The model under review builds one solid part; all positions refer to its coordinate system, in mm. A direction names the side the tool comes from. Round coordinates to 2 decimals unless told otherwise and drop trailing zeros. Write each loop counter-clockwise with the first axis right and the second up, starting at its lowest first coordinate (ties: lowest second). Pieces come first, ordered by that corner, then holes. Notation, with made-up numbers: (30, 4.25) - (64, 4.25) arc R25 ccw to (64, 27.25) - close; hole circle Ø7 at (65.5, 42). An arc over 180 degrees is marked (long way). Return JSON: item names as keys, results as strings.
from build123d import *

# Parameters (mm, degrees)
BOSS_EXTRUDE1_DEPTH = 3
SKETCH2_R           = 17
BOSS_EXTRUDE2_DEPTH = 5.5
SKETCH5_R           = 14
BOSS_EXTRUDE3_DEPTH = 3.5
SKETCH6_R           = 11
CUT_EXTRUDE1_DEPTH  = 44.5
SKETCH7_R           = 2.5
CUT_EXTRUDE2_DEPTH  = 44.5
SKETCH8_R           = 2.5
CUT_EXTRUDE3_DEPTH  = 44.5
SKETCH9_R           = 2.5
CUT_EXTRUDE4_DEPTH  = 44.5
SKETCH10_R          = 2.5
CUT_EXTRUDE5_DEPTH  = 44.5
FILLET23_R          = 2


with BuildPart() as part:
    # Sketch1 → Boss-Extrude1 (new body)
    with BuildSketch(Plane(origin=(0, 0, 0), x_dir=(1, 0, 0), z_dir=(0, 1, 0))):
        with BuildLine():
            ThreePointArc((-12.368882592, -22.86942814), (-2.248386141, -25.902601409), (8.243375366, -24.65860423))
            ThreePointArc((8.243375366, -24.65860423), (11.092172188, -24.325815059), (13.835297391, -25.163464204))
            ThreePointArc((13.835297391, -25.163464204), (20.585915101, -24.499389777), (22.403221797, -17.964159812))
            ThreePointArc((22.403221797, -17.964159812), (22.050754674, -15.117730664), (22.86942814, -12.368882592))
            ThreePointArc((22.86942814, -12.368882592), (25.902601409, -2.248386141), (24.65860423, 8.243375366))
            ThreePointArc((24.65860423, 8.243375366), (24.325815059, 11.092172188), (25.163464204, 13.835297391))
            ThreePointArc((25.163464204, 13.835297391), (24.499389777, 20.585915101), (17.964159812, 22.403221797))
            ThreePointArc((17.964159812, 22.403221797), (15.117730664, 22.050754674), (12.368882592, 22.86942814))
            ThreePointArc((12.368882592, 22.86942814), (2.248386141, 25.902601409), (-8.243375366, 24.65860423))
            ThreePointArc((-8.243375366, 24.65860423), (-11.092172188, 24.325815059), (-13.835297391, 25.163464204))
            ThreePointArc((-13.835297391, 25.163464204), (-20.585915101, 24.499389777), (-22.403221797, 17.964159812))
            ThreePointArc((-22.403221797, 17.964159812), (-22.050754674, 15.117730664), (-22.86942814, 12.368882592))
            ThreePointArc((-22.86942814, 12.368882592), (-25.902601409, 2.248386141), (-24.65860423, -8.243375366))
            ThreePointArc((-24.65860423, -8.243375366), (-24.325815059, -11.092172188), (-25.163464204, -13.835297391))
            ThreePointArc((-25.163464204, -13.835297391), (-24.499389777, -20.585915101), (-17.964159812, -22.403221797))
            ThreePointArc((-17.964159812, -22.403221797), (-15.117730664, -22.050754674), (-12.368882592, -22.86942814))
        make_face()
    extrude(amount=-BOSS_EXTRUDE1_DEPTH)

    # Sketch2 → Boss-Extrude2 (add)
    with BuildSketch(Plane(origin=(0, 0, 0), x_dir=(1, 0, 0), z_dir=(0, 1, 0))):
        with Locations(Location((0, 0, 0), (0, 0, 270))):
            Circle(SKETCH2_R)
    extrude(amount=BOSS_EXTRUDE2_DEPTH)

    # Sketch5 → Boss-Extrude3 (add)
    with BuildSketch(Plane(origin=(0, 5.5, 0), x_dir=(1, 0, 0), z_dir=(0, 1, 0))):
        with Locations(Location((0, 0, 0), (0, 0, 270))):
            Circle(SKETCH5_R)
    extrude(amount=BOSS_EXTRUDE3_DEPTH)

    # Sketch6 → Cut-Extrude1 (cut)
    with BuildSketch(Plane(origin=(0, 9, 0), x_dir=(1, 0, 0), z_dir=(0, 1, 0))):
        with Locations(Location((0, 0, 0), (0, 0, 270))):
            Circle(SKETCH6_R)
    extrude(amount=-CUT_EXTRUDE1_DEPTH, mode=Mode.SUBTRACT)

    # Sketch7 → Cut-Extrude2 (cut)
    with BuildSketch(Plane(origin=(0, 0, 0), x_dir=(1, 0, 0), z_dir=(0, 1, 0))):
        with Locations(Location((-16.72605602, 19.905754194, 0), (0, 0, 270))):
            Circle(SKETCH7_R)
    extrude(amount=-CUT_EXTRUDE2_DEPTH, mode=Mode.SUBTRACT)

    # Sketch8 → Cut-Extrude3 (cut)
    with BuildSketch(Plane(origin=(0, 0, 0), x_dir=(1, 0, 0), z_dir=(0, 1, 0))):
        with Locations(Location((16.72605602, -19.905754194, 0), (0, 0, 270))):
            Circle(SKETCH8_R)
    extrude(amount=-CUT_EXTRUDE3_DEPTH, mode=Mode.SUBTRACT)

    # Sketch9 → Cut-Extrude4 (cut)
    with BuildSketch(Plane(origin=(0, 0, 0), x_dir=(1, 0, 0), z_dir=(0, 1, 0))):
        with Locations(Location((-19.905754194, -16.72605602, 0), (0, 0, 270))):
            Circle(SKETCH9_R)
    extrude(amount=-CUT_EXTRUDE4_DEPTH, mode=Mode.SUBTRACT)

    # Sketch10 → Cut-Extrude5 (cut)
    with BuildSketch(Plane(origin=(0, 0, 0), x_dir=(1, 0, 0), z_dir=(0, 1, 0))):
        with Locations(Location((19.905754194, 16.72605602, 0), (0, 0, 270))):
            Circle(SKETCH10_R)
    extrude(amount=-CUT_EXTRUDE5_DEPTH, mode=Mode.SUBTRACT)

    # Fillet23
    fillet23_edges = [part.edges().sort_by_distance(p)[0] for p in [
        (0, 0, -17),
    ]]
    fillet(fillet23_edges, radius=FILLET23_R)


solid = part.part
(1) Add section A-A (z = 0). Write out the cut boundary in (x, y).
Filled in:
{"outline": "(-26, -3) - (-11, -3) - (-11, 9) - (-14, 9) - (-14, 5.5) - (-17, 5.5) - (-17, 2) arc R2 cw to (-19, 0) - (-26, 0) - close; (11, -3) - (26, -3) - (26, 0) - (19, 0) arc R2 cw to (17, 2) - (17, 5.5) - (14, 5.5) - (14, 9) - (11, 9) - close"}
(2) Add section D-D (z = 20). Write out the cut boundary in (x, y).
Filled in:
{"outline": "(-24.93, -3) - (14.23, -3) - (14.23, 0) - (-24.93, 0) - close; (19.22, -3) - (22.73, -3) - (22.73, 0) - (19.22, 0) - close"}
(3) Add section B-B (x = 0). Write out the cut boundary in (y, z).
Filled in:
{"outline": "(-3, -26) - (0, -26) - (0, -19) arc R2 cw to (2, -17) - (5.5, -17) - (5.5, -14) - (9, -14) - (9, -11) - (-3, -11) - close; (-3, 11) - (9, 11) - (9, 14) - (5.5, 14) - (5.5, 17) - (2, 17) arc R2 cw to (0, 19) - (0, 26) - (-3, 26) - close"}
(4) Add section C-C (y = 8.25). Write out the cut boundary in (x, z).
Filled in:
{"outline": "circle Ø28 at (0, 0); hole circle Ø22 at (0, 0)"}
(5) For faces 4 (the cylindrical face through (18.834, -1.479, 21.25)), 5 (the flat face through (13, 5.5, -6)), list the 3-axis set-ups (+Z, -Z, +X, -X, +Y, -Y) from which the entire face can be reached by the end or side of a thin tool; tool diameter is ignored.
Filled in:
{"face 4": "+Y, -Y", "face 5": "+Y"}
(6) Clearance check with flat-ended pins moving along their axes: pin 1 Ø1 at (x, y) = (-5.5, 0) entering from -Z; pin 2 Ø6.5 at (x, z) = (-19.91, 16.73) entering from +Y; pin 3 Ø1.5 at (y, z) = (6.5, -11) entering from -X. State where each tip first meets the part, or that it passes through.
Filled in:
{"pin 1": "stops at z = -25.51", "pin 2": "stops at y = 0", "pin 3": "stops at x = -9.54"}
(7) Wall thickness on line 1 (Y direction, x = 23, z = 11); line 2 (X direction, y = 7.75, z = -10); line 3 (X direction, y = 7.75, z = 2): over which ranges is each line inside the solid? List them lowest first.
Filled in:
{"line 1": "y = -3 to 0", "line 2": "x = -9.8 to -4.58, 4.58 to 9.8", "line 3": "x = -13.86 to -10.82, 10.82 to 13.86"}
(8) Mouldability with a two-part tool opening along X and no side actions: class faces 1 (the flat face through (-9.3, 9, 6.2)), 2 (the cylindrical face through (22.048, -1.479, 15.158)), 3 (the cylindrical face through (15.158, -1.479, -22.048)) as released by +X, released by -X, zero draft, split by the parting line, or undercut.
Filled in:
{"face 1": "zero draft", "face 2": "released by +X", "face 3": "undercut"}
